from build123d import *

# Parameters (mm, degrees)
SKETCH1_R           = 2.2
BOSS_EXTRUDE1_DEPTH = 5
BOSS_EXTRUDE2_START = 5
SKETCH1_3_W         = 4.6228
SKETCH1_3_H         = 4.6228
BOSS_EXTRUDE2_DEPTH = 2
FILLET1_R           = 3
FILLET2_R           = 0.508
FILLET3_R           = 0.5


with BuildPart() as part:
    # Sketch1 → Boss-Extrude1 (new body)
    with BuildSketch(Plane(origin=(0, 0, 0), x_dir=(1, 0, 0), z_dir=(0, 1, 0))):
        Polygon((-80.7, 4.5), (-71.7, 4.5), (-71.7, -23.15), (-4.5, -23.15), (-4.5, 4.5), (4.5, 4.5), (4.5, -55.3), (-4.5, -55.3), (-80.7, -29.9), align=None)
        with Locations(Location((0, 0, 0), (0, 0, 270))):
            Circle(SKETCH1_R, mode=Mode.SUBTRACT)
        with Locations(Location((-76.2, 0, 0), (0, 0, 270))):
            Circle(SKETCH1_R, mode=Mode.SUBTRACT)
        with Locations(Location((0, -50.8, 0), (0, 0, 270))):
            Circle(SKETCH1_R, mode=Mode.SUBTRACT)
        Polygon((-70.138611699, -28.15), (-4.5, -28.15), (-4.5, -50.029537233), align=None, mode=Mode.SUBTRACT)
    extrude(amount=BOSS_EXTRUDE1_DEPTH)

    # Sketch1<3> → Boss-Extrude2 (add)
    with BuildSketch(Plane(origin=(0, 0, 0), x_dir=(1, 0, 0), z_dir=(0, 1, 0)).offset(BOSS_EXTRUDE2_START)):
        with Locations((-76.2, -25.4)):
            Rectangle(SKETCH1_3_W, SKETCH1_3_H)
        with Locations((0, -25.4)):
            Rectangle(SKETCH1_3_W, SKETCH1_3_H)
    extrude(amount=BOSS_EXTRUDE2_DEPTH)

    # Fillet1
    fillet1_edges = [part.edges().sort_by_distance(p)[0] for p in [
        (-4.5, 2.5, 28.15),
        (-4.5, 2.5, 50.029537233),
        (-80.7, 2.5, -4.5),
        (-71.7, 2.5, -4.5),
        (-71.7, 2.5, 23.15),
        (-4.5, 2.5, 23.15),
        (-4.5, 2.5, -4.5),
        (4.5, 2.5, -4.5),
        (4.5, 2.5, 55.3),
        (-4.5, 2.5, 55.3),
        (-80.7, 2.5, 29.9),
    ]]
    fillet(fillet1_edges, radius=FILLET1_R)

    # Fillet2
    fillet2_edges = [part.edges().sort_by_distance(p)[0] for p in [
        (-78.5114, 6, 23.0886),
        (-76.2, 7, 27.7114),
        (-78.5114, 6, 27.7114),
        (-73.8886, 7, 25.4),
        (-73.8886, 6, 27.7114),
        (-73.8886, 6, 23.0886),
        (-78.5114, 7, 25.4),
        (-76.2, 7, 23.0886),
        (-2.3114, 6, 23.0886),
        (0, 7, 27.7114),
        (-2.3114, 6, 27.7114),
        (2.3114, 7, 25.4),
        (2.3114, 6, 27.7114),
        (2.3114, 6, 23.0886),
        (-2.3114, 7, 25.4),
        (0, 7, 23.0886),
    ]]
    fillet(fillet2_edges, radius=FILLET2_R)

    # Fillet3
    fillet3_edges = [part.edges().sort_by_distance(p)[0] for p in [
        (-70.138611699, 2.5, 28.15),
    ]]
    fillet(fillet3_edges, radius=FILLET3_R)


solid = part.part
For this review, take the finished solid that the model builds, in its own axes (mm). A direction names the side the tool comes from. Round coordinates to 2 decimals unless told otherwise and drop trailing zeros. Write each loop counter-clockwise with the first axis right and the second up, starting at its lowest first coordinate (ties: lowest second). Pieces come first, ordered by that corner, then holes. Notation, with made-up numbers: M 81.25,66 L 136.25,66 A21 ccw 136.25,87 Z; hole C -39.5,-2 d8. An arc over 180 degrees is marked long. Write item = value, one per line. Start each with the question number.
(1) We need section C-C (x = -76.2). Give the boundary of the cut face in (y, z), then the cut area to 3 significant figures.
(2) We need section D-D (y = 1). Give the boundary of the cut face in (x, z).
(3) We need section B-B (z = 0). Give the boundary of the cut face in (x, y), then the cut area to 3 significant figures.
(4) The part is to be moulded in two halves that separate along Z. For faces 1 (the face through (-41.289, 2.465, 43.037)), 2 (the face through (0, 7, 25)), 3 (the face through (-5.4, 2.54, 29.01)), say which applies: +Z half, -Z half, draft (parallel to the pull), parting line (faces both ways), or undercut.
(5) We need section A-A (z = 50.8). Give the boundary of the cut face in (x, y).
(6) For line 1 along X through (y, z) = (1.05, 0); line 2 along X through (y, z) = (3.5, 3.5); line 3 along Y through (x, z) = (-73, 30), list the stretches that pass through material, from the lowest coordinate up.
(7) For faces 4 (the face through (4.5, 2, 25)), 5 (the face through (-5.4, 2.54, 22.29)), 6 (the face through (-5.714, 2.535, 48.278)), list the 3-axis set-ups (+Z, -Z, +X, -X, +Y, -Y) from which the entire face can be reached by the end or side of a thin tool; tool diameter is ignored.
(8) Clearance check with flat-ended pins moving along their axes: pin 1 Ø7 at (x, z) = (-76.2, 0) entering from +Y; pin 2 Ø4 at (x, y) = (-32.5, 2.5) entering from +Z; pin 3 Ø1.2 at (x, y) = (-77, 6) entering from -Z; pin 4 Ø8 at (x, z) = (-34, 19) entering from +Y. State where each tip first meets the part, or that it passes through.
Results found:
q1.outline = M 0,-4.5 L 5,-4.5 L 5,-2.2 L 0,-2.2 Z; M 0,2.2 L 5,2.2 L 5,23.09 L 6.49,23.09 A0.51 ccw 7,23.6 L 7,27.2 A0.51 ccw 6.49,27.71 L 5,27.71 L 5,31.4 L 0,31.4 Z
q1.area = 167 mm²
q2.outline = M -80.7,-1.5 A3 ccw -77.7,-4.5 L -74.7,-4.5 A3 ccw -71.7,-1.5 L -71.7,20.15 A3 cw -68.7,23.15 L -7.5,23.15 A3 cw -4.5,20.15 L -4.5,-1.5 A3 ccw -1.5,-4.5 L 1.5,-4.5 A3 ccw 4.5,-1.5 L 4.5,52.3 A3 ccw 1.5,55.3 L -4.01,55.3 A3 ccw -4.96,55.15 L -78.65,30.58 A3 ccw -80.7,27.74 Z; hole C -76.2,0 d4.4; hole M -67.22,29.12 A0.5 ccw -67.06,28.15 L -7.5,28.15 A3 ccw -4.5,31.15 L -4.5,45.87 A3 ccw -8.45,48.71 Z; hole C 0,0 d4.4; hole C 0,50.8 d4.4
q3.outline = M -80.7,0 L -78.4,0 L -78.4,5 L -80.7,5 Z; M -74,0 L -71.7,0 L -71.7,5 L -74,5 Z; M -4.5,0 L -2.2,0 L -2.2,5 L -4.5,5 Z; M 2.2,0 L 4.5,0 L 4.5,5 L 2.2,5 Z
q3.area = 46.0 mm²
q4.face_1 = +Z half
q4.face_2 = draft
q4.face_3 = undercut
q5.outline = M -18,0 L -2.2,0 L -2.2,5 L -18,5 Z; M 2.2,0 L 4.5,0 L 4.5,5 L 2.2,5 Z
q6.line_1 = -80.7 to -78.4, -74 to -71.7, -4.5 to -2.2, 2.2 to 4.5
q6.line_2 = -80.7 to -71.7, -4.5 to 4.5
q6.line_3 = 0 to 5
q7.face_4 = +Z, -Z, +X, +Y, -Y
q7.face_5 = -Z, +Y, -Y
q7.face_6 = +Y, -Y
q8.pin_1 = 5
q8.pin_2 = 46.63
q8.pin_3 = 23.09
q8.pin_4 = through
